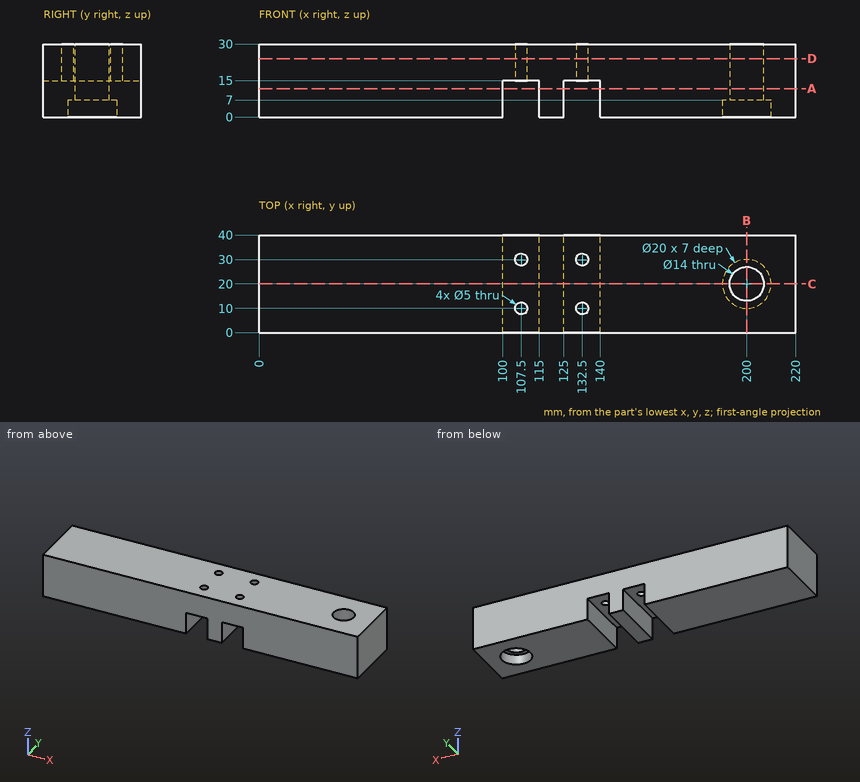
Design review of the part shown in the three views and the two pictorial views. Dimensions are in mm from the part's minimum x, y and z. Give positions to 0.01 mm unless a question says otherwise; leave off trailing zeros. Loops run counter-clockwise (first coordinate to the right, second up) from the corner with the lowest first, then second, coordinate; pieces in that order, holes last. Notation, with made-up numbers: (-20, 60.5) - (34, 60.5) arc R16 cw to (34, 79.5) - close; hole circle Ø9 at (-15, 89). An arc over 180 degrees is marked (long way). Use CSV: the item, a comma, the result in double quotes. Start each with the question number.
1. Add section C-C (y = 20). State the section outline as (x, z) points, plus the area to 3 significant figures.
2. Add section D-D (z = 24). State the section outline as (x, y) points, plus the area to 3 significant figures.
3. Add section A-A (z = 11.75). State the section outline as (x, y) points, plus the area to 3 significant figures.
4. Add section B-B (x = 200). State the section outline as (y, z) points, plus the area to 3 significant figures.
5. Wall thickness on L1, parallel to Y at x = 200, z = 22; L2, parallel to Y at x = 132.5, z = 21.75; L3, parallel to X at y = 22, z = 9.25: over which ranges is each line inside the solid? List them lowest first.
6. Insertion check: P1, Ø16.5, axis at x = 107, y = 23, coming from the -Z side; P2, Ø10, axis at x = 200, y = 23, coming from the -Z side; P3, Ø12, axis at x = 133.5, y = 17, coming from the -Z side. Each pin has a flat end and moves straight along its axis. Give the tip position at first contact, or say it passes through.
Results found:
1,outline,"(0, 0) - (100, 0) - (100, 15) - (115, 15) - (115, 0) - (125, 0) - (125, 15) - (140, 15) - (140, 0) - (190, 0) - (190, 7) - (193, 7) - (193, 30) - (0, 30) - close; (207, 7) - (210, 7) - (210, 0) - (220, 0) - (220, 30) - (207, 30) - close"
1,area,"5,690 mm²"
2,outline,"(0, 0) - (220, 0) - (220, 40) - (0, 40) - close; hole circle Ø5 at (107.5, 10); hole circle Ø5 at (107.5, 30); hole circle Ø5 at (132.5, 10); hole circle Ø5 at (132.5, 30); hole circle Ø14 at (200, 20)"
2,area,"8,570 mm²"
3,outline,"(0, 0) - (100, 0) - (100, 40) - (0, 40) - close; (115, 0) - (125, 0) - (125, 40) - (115, 40) - close; (140, 0) - (220, 0) - (220, 40) - (140, 40) - close; hole circle Ø14 at (200, 20)"
3,area,"7,450 mm²"
4,outline,"(0, 0) - (10, 0) - (10, 7) - (13, 7) - (13, 30) - (0, 30) - close; (27, 7) - (30, 7) - (30, 0) - (40, 0) - (40, 30) - (27, 30) - close"
4,area,"738 mm²"
5,L1,"y = 0 to 13, 27 to 40"
5,L2,"y = 0 to 7.5, 12.5 to 27.5, 32.5 to 40"
5,L3,"x = 0 to 100, 115 to 125, 140 to 193.29, 206.71 to 220"
6,P1,"stops at z = 0"
6,P2,"stops at z = 7"
6,P3,"stops at z = 15"
